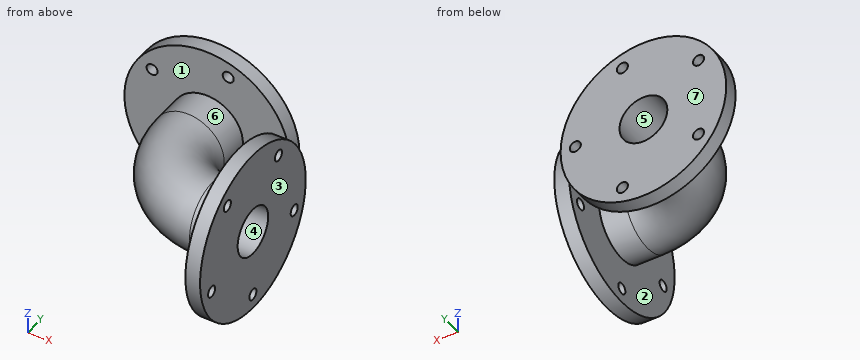
from build123d import *

# Parameters (mm, degrees)
SKETCH2_R           = 48.5
SKETCH3_R           = 112.5
BOSS_EXTRUDE1_DEPTH = 20
SKETCH4_R           = 112.5
BOSS_EXTRUDE2_DEPTH = 20
SKETCH5_R           = 32.5
SKETCH6_R           = 7.5
CUT_EXTRUDE1_DEPTH  = 30
SKETCH7_R           = 7.5
CUT_EXTRUDE3_DEPTH  = 30


with BuildPart() as part:
    # Sweep1: sweep along a path in Sketch1
    with BuildLine(Plane.XY) as sweep1_path:
        Line((0, 0), (-55, 0))
        ThreePointArc((-55, 0), (-118.639610307, 26.360389693), (-145, 90))
        Line((-145, 90), (-145, 150))
    # Sketch2 → Sweep1 (sweep)
    with BuildSketch(Plane(origin=(0, 0, 0), x_dir=(0, 0, -1), z_dir=(1, 0, 0))):
        Circle(SKETCH2_R)
    sweep(path=sweep1_path.line)

    # Sketch3 → Boss-Extrude1 (add)
    with BuildSketch(Plane(origin=(0, 0, 0), x_dir=(0, 0, -1), z_dir=(1, 0, 0))):
        Circle(SKETCH3_R)
    extrude(amount=-BOSS_EXTRUDE1_DEPTH)

    # Sketch4 → Boss-Extrude2 (add)
    with BuildSketch(Plane(origin=(0, 150, 0), x_dir=(1, 0, 0), z_dir=(0, 1, 0))):
        with Locations((-145, 0)):
            Circle(SKETCH4_R)
    extrude(amount=-BOSS_EXTRUDE2_DEPTH)

    # Cut-Sweep1: sweep along a path in Sketch1<2>
    with BuildLine(Plane.XY) as cut_sweep1_path:
        Line((0, 0), (-55, 0))
        ThreePointArc((-55, 0), (-118.639610307, 26.360389693), (-145, 90))
        Line((-145, 90), (-145, 150))
    # Sketch5 → Cut-Sweep1 (sweep, cut)
    with BuildSketch(Plane(origin=(0, 0, 0), x_dir=(0, 0, -1), z_dir=(1, 0, 0))):
        Circle(SKETCH5_R)
    sweep(path=cut_sweep1_path.line, mode=Mode.SUBTRACT)

    # Sketch6 → Cut-Extrude1 (cut)
    with BuildSketch(Plane(origin=(0, 150, 0), x_dir=(1, 0, 0), z_dir=(0, 1, 0))):
        with Locations((-52.5, 0)):
            Circle(SKETCH6_R)
        with Locations((-116.41592802, -87.972727757)):
            Circle(SKETCH6_R)
        with Locations((-219.83407198, -54.370135837)):
            Circle(SKETCH6_R)
        with Locations((-219.83407198, 54.370135837)):
            Circle(SKETCH6_R)
        with Locations((-116.41592802, 87.972727757)):
            Circle(SKETCH6_R)
    extrude(amount=-CUT_EXTRUDE1_DEPTH, mode=Mode.SUBTRACT)

    # Sketch7 → Cut-Extrude3 (cut)
    with BuildSketch(Plane(origin=(0, 0, 0), x_dir=(0, 0, -1), z_dir=(1, 0, 0))):
        with Locations((92.5, 0)):
            Circle(SKETCH7_R)
        with Locations((28.58407198, -87.972727757)):
            Circle(SKETCH7_R)
        with Locations((-74.83407198, -54.370135837)):
            Circle(SKETCH7_R)
        with Locations((-74.83407198, 54.370135837)):
            Circle(SKETCH7_R)
        with Locations((28.58407198, 87.972727757)):
            Circle(SKETCH7_R)
    extrude(amount=-CUT_EXTRUDE3_DEPTH, mode=Mode.SUBTRACT)


solid = part.part
The listing builds one solid part. Answer for the finished solid, in the listing's coordinates (mm). Face numbers are marked on the shaded views. A direction names the side the tool comes from. Give positions to 0.01 mm unless a question says otherwise; leave off trailing zeros. Write each loop counter-clockwise with the first axis right and the second up, starting at its lowest first coordinate (ties: lowest second). Pieces come first, ordered by that corner, then holes. Notation, with made-up numbers: (74, -17) -> (107, -17) arc R30 ccw to (107, 17) -> close; hole circle Ø10 at (5, 72). An arc over 180 degrees is marked (long way). Use a Markdown table: item, result.
(1) For the marked faces 4, 5, 6 and 7, determine the directions among +Z, -Z, +X, -X, +Y, -Y from which every point of the face is accessible in a straight line to the end or side of a thin tool.
Return value:
| item | result |
|---|---|
| face 4 | +X |
| face 5 | +Y |
| face 6 | none |
| face 7 | +Z, -Z, +X, -X, +Y |
(2) Find the intervals of material crossed by probe 1 along X at (y, z) = (138, 0); probe 2 along Y at (x, z) = (-27, 0); probe 3 along X at (y, z) = (68.5, -25), in increasing order. Write a range as from..to.
Return value:
| item | result |
|---|---|
| probe 1 | -257.5..-177.5, -112.5..-60, -45..-32.5 |
| probe 2 | -48.5..-32.5, 32.5..48.5 |
| probe 3 | -184.79..-163.66, -120.81..-98.41, -20..0 |
(3) Section C-C, the plane x = -90.5 is taken. Give the number of separate pieces and of enclosed holes in the cut face, then the cut area to 3 significant figures.
Return value:
| item | result |
|---|---|
| separate pieces | 2 |
| enclosed holes | 1 |
| area | 8,660 mm2 |
(4) Determine the mould class of the marked faces 1, 2 and 3 for opening direction X: released by +X, released by -X, zero draft, split by the parting line, or undercut.
Return value:
| item | result |
|---|---|
| face 1 | zero draft |
| face 2 | undercut |
| face 3 | released by +X |
(5) Section B-B, the plane y = 133.5 is taken. Determine the outline of the cut face in (x, z), then the cut area to 3 significant figures.
Return value:
| item | result |
|---|---|
| outline | circle Ø225 at (-145, 0); hole circle Ø15 at (-219.83, -54.37); hole circle Ø15 at (-219.83, 54.37); hole circle Ø65 at (-145, 0); hole circle Ø15 at (-116.42, -87.97); hole circle Ø15 at (-116.42, 87.97); hole circle Ø15 at (-52.5, 0) |
| area | 35,600 mm2 |
(6) Section A-A, the plane z = 0 is taken. Determine the outline of the cut face in (x, y).
Return value:
| item | result |
|---|---|
| outline | (-257.5, 130) -> (-193.5, 130) -> (-193.5, 90) arc R138.5 ccw to (-55, -48.5) -> (-20, -48.5) -> (-20, -112.5) -> (0, -112.5) -> (0, -32.5) -> (-55, -32.5) arc R122.5 cw to (-177.5, 90) -> (-177.5, 150) -> (-257.5, 150) -> close; (-112.5, 90) arc R57.5 ccw to (-55, 32.5) -> (0, 32.5) -> (0, 112.5) -> (-20, 112.5) -> (-20, 48.5) -> (-55, 48.5) arc R41.5 cw to (-96.5, 90) -> (-96.5, 130) -> (-60, 130) -> (-60, 150) -> (-112.5, 150) -> close; (-45, 130) -> (-32.5, 130) -> (-32.5, 150) -> (-45, 150) -> close |
(7) Flat-ended cylindrical pins translate along their axes: P1, Ø1, axis at x = -82, z = 75, coming from the -Y side; P2, Ø9, axis at x = -52.5, z = 0, coming from the +Y side; P3, Ø1, axis at y = 72.5, z = -82.5, coming from the -X side. Find the tip coordinate at first contact, or state that the pin passes through.
Return value:
| item | result |
|---|---|
| P1 | y = 130 |
| P2 | y = 48.55 |
| P3 | x = -20 |
